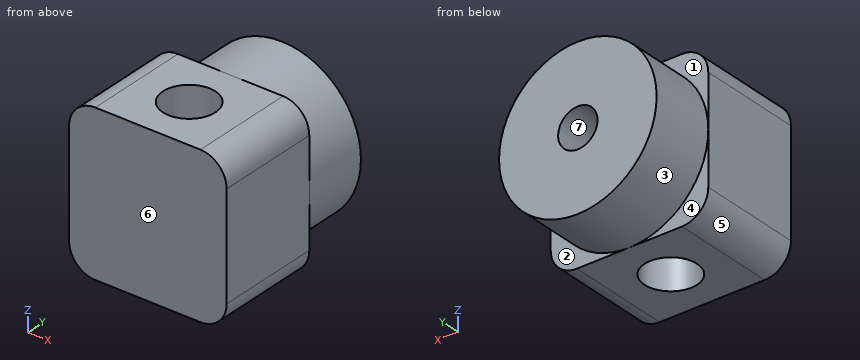
from build123d import *

# Parameters (mm, degrees)
SKETCH_1_R          = 6
EXTRUDE_1_DEPTH     = 5
SKETCH_2_W          = 12
SKETCH_2_H          = 12
EXTRUDE_2_DEPTH     = 8
FILLET_1_R          = 2
SKETCH_3_R          = 1.5
CUT_EXTRUDE_1_DEPTH = 5
SKETCH_4_R          = 2
CUT_EXTRUDE_2_DEPTH = 16.620499352


with BuildPart() as part:
    # 草图1 → 凸台-拉伸1 (new body)
    with BuildSketch(Plane(origin=(0, 0, 0), x_dir=(1, 0, 0), z_dir=(0, 1, 0))):
        with Locations(Location((0, 0, 0), (0, 0, 270))):
            Circle(SKETCH_1_R)
    extrude(amount=EXTRUDE_1_DEPTH)

    # 草图2 → 凸台-拉伸2 (add)
    with BuildSketch(Plane.XZ):
        Rectangle(SKETCH_2_W, SKETCH_2_H)
    extrude(amount=EXTRUDE_2_DEPTH)

    # 圆角1
    fillet_1_edges = [part.edges().sort_by_distance(p)[0] for p in [
        (-6, -4, 6),
        (-6, -4, -6),
        (6, -4, -6),
        (6, -4, 6),
    ]]
    fillet(fillet_1_edges, radius=FILLET_1_R)

    # 草图3 → 切除-拉伸1 (cut)
    with BuildSketch(Plane(origin=(0, 5, 0), x_dir=(1, 0, 0), z_dir=(0, 1, 0))):
        with Locations(Location((0, 0, 0), (0, 0, 270))):
            Circle(SKETCH_3_R)
    extrude(amount=-CUT_EXTRUDE_1_DEPTH, mode=Mode.SUBTRACT)

    # 草图4 → 切除-拉伸2 (cut, through all)
    with BuildSketch(Plane(origin=(0, 0, -6), x_dir=(-1, 0, 0), z_dir=(0, 0, -1))):
        with Locations((0, -4)):
            Circle(SKETCH_4_R)
    extrude(amount=-CUT_EXTRUDE_2_DEPTH, mode=Mode.SUBTRACT)


solid = part.part
Read the model definition and answer for the solid it produces. Units are mm, in the model's axes. Face numbers are marked on the shaded views. A direction names the side the tool comes from. Coordinates: 2 decimals unless noted, no trailing zeros. Loops run counter-clockwise (first coordinate to the right, second up) from the corner with the lowest first, then second, coordinate; pieces in that order, holes last. Notation, with made-up numbers: (-18.75, 31) -> (6.25, 31) arc R15 ccw to (6.25, 35) -> close; hole circle Ø1 at (23, 13.5). An arc over 180 degrees is marked (long way). Answer in a Markdown table with one row per item.
Item 1: For the marked faces 1, 2, 3 and 4, determine the directions among +Z, -Z, +X, -X, +Y, -Y from which every point of the face is accessible in a straight line to the end or side of a thin tool.
Returned:
| item | result |
|---|---|
| face 1 | +Z, -X, +Y |
| face 2 | -Z, +X, +Y |
| face 3 | +Y |
| face 4 | -Z, -X, +Y |
Item 2: For a pull along Z with two mould halves and no side action, classify the marked faces 5, 6 and 7 as released by +Z, released by -Z, zero draft, split by the parting line, or undercut.
Returned:
| item | result |
|---|---|
| face 5 | released by -Z |
| face 6 | zero draft |
| face 7 | undercut |
Item 3: Straight lines are drawn through the part: line 1 along Y through (x, z) = (0, 0.75); line 2 along Y through (x, z) = (0, 3.5); line 3 along X through (y, z) = (-5, 2.5). For each, find the intervals that lie inside material, in ascending order. Write a range as [from, to].
Returned:
| item | result |
|---|---|
| line 1 | y = [-8, -6], [-2, 0] |
| line 2 | y = [-8, -6], [-2, 5] |
| line 3 | x = [-6, -1.73], [1.73, 6] |
Item 4: A cutting plane is placed at B-B on x = 1.75. Determine the outline of the cut face in (y, z).
Returned:
| item | result |
|---|---|
| outline | (-8, -6) -> (-4.97, -6) -> (-4.97, 6) -> (-8, 6) -> close; (-3.03, -6) -> (0, -6) -> (0, -5.74) -> (5, -5.74) -> (5, 5.74) -> (0, 5.74) -> (0, 6) -> (-3.03, 6) -> close |
Item 5: Each of these flat-tipped pins is pushed along its axis until it touches: P1, Ø1, axis at x = 2, y = 1, coming from the -Z side; P2, Ø0.9, axis at x = -0.5, z = -0.5, coming from the +Y side. Where does it stop, or does it pass through?
Returned:
| item | result |
|---|---|
| P1 | stops at z = -5.81 |
| P2 | stops at y = 0 |
Item 6: A cutting plane is placed at A-A on y = -4. Determine the outline of the cut face in (x, z), plus the area to 3 significant figures.
Returned:
| item | result |
|---|---|
| outline | (-6, -4) arc R2 ccw to (-4, -6) -> (-2, -6) -> (-2, 6) -> (-4, 6) arc R2 ccw to (-6, 4) -> close; (2, -6) -> (4, -6) arc R2 ccw to (6, -4) -> (6, 4) arc R2 ccw to (4, 6) -> (2, 6) -> close |
| area | 92.6 mm^2 |
Item 7: A cutting plane is placed at C-C on z = 2.5. Determine the outline of the cut face in (x, y), plus the area to 3 significant figures.
Returned:
| item | result |
|---|---|
| outline | (-6, -8) -> (6, -8) -> (6, 0) -> (5.45, 0) -> (5.45, 5) -> (-5.45, 5) -> (-5.45, 0) -> (-6, 0) -> close; hole circle Ø4 at (0, -4) |
| area | 138 mm^2 |
Item 8: A cutting plane is placed at D-D on y = 2.75. Determine the outline of the cut face in (x, z), plus the area to 3 significant figures.
Returned:
| item | result |
|---|---|
| outline | circle Ø12 at (0, 0); hole circle Ø3 at (0, 0) |
| area | 106 mm^2 |
